```python
from build123d import *

# Parameters (mm, degrees)
SKETCH_1_R          = 15
EXTRUDE_1_DEPTH     = 20
SKETCH_10_R         = 10
EXTRUDE_10_DEPTH    = 14
SKETCH_11_R         = 10
EXTRUDE_11_DEPTH    = 14
SKETCH_12_W         = 12
SKETCH_12_H         = 50
EXTRUDE_12_DEPTH    = 10
SKETCH_13_W         = 80
SKETCH_13_H         = 12
EXTRUDE_13_DEPTH    = 10
SKETCH_14_R         = 5
CUT_EXTRUDE_1_DEPTH = 111
SKETCH_15_R         = 4
CUT_EXTRUDE_2_DEPTH = 111
SKETCH_16_R         = 7
CUT_EXTRUDE_3_DEPTH = 111
SKETCH_17_W         = 3
SKETCH_17_H         = 4
CUT_EXTRUDE_4_DEPTH = 111


with BuildPart() as part:
    # Sketch 1 → Extrude 1 (new body)
    with BuildSketch(Plane.XY.offset(-10)):
        Circle(SKETCH_1_R)
    extrude(amount=EXTRUDE_1_DEPTH)



with BuildPart() as body_2:
    # Sketch 10 → Extrude 10 (new body)
    with BuildSketch(Plane.XY.offset(-10)):
        with Locations((0, 50)):
            Circle(SKETCH_10_R)
    extrude(amount=EXTRUDE_10_DEPTH)


with BuildPart() as body_3:
    # Sketch 11 → Extrude 11 (new body)
    with BuildSketch(Plane.XY.offset(-10)):
        with Locations((80, 0)):
            Circle(SKETCH_11_R)
    extrude(amount=EXTRUDE_11_DEPTH)


with BuildPart() as part_1:
    add(part.part)

    add(body_2.part)  # Extrude 12 merges body 2
    # Sketch 12 → Extrude 12 (add)
    with BuildSketch(Plane.XY.offset(-10)):
        with Locations((0, 25)):
            Rectangle(SKETCH_12_W, SKETCH_12_H)
    extrude(amount=EXTRUDE_12_DEPTH)


    add(body_3.part)  # Extrude 13 merges body 3
    # Sketch 13 → Extrude 13 (add)
    with BuildSketch(Plane.XY.offset(-10)):
        with Locations((40, 0)):
            Rectangle(SKETCH_13_W, SKETCH_13_H)
    extrude(amount=EXTRUDE_13_DEPTH)

    # Sketch 14 → Cut-Extrude 1 (cut, through all)
    with BuildSketch(Plane.XY.offset(-10)):
        with Locations((0, 50)):
            Circle(SKETCH_14_R)
    extrude(amount=CUT_EXTRUDE_1_DEPTH, mode=Mode.SUBTRACT)

    # Sketch 15 → Cut-Extrude 2 (cut, through all)
    with BuildSketch(Plane.XY.offset(-10)):
        with Locations((80, 0)):
            Circle(SKETCH_15_R)
    extrude(amount=CUT_EXTRUDE_2_DEPTH, mode=Mode.SUBTRACT)

    # Sketch 16 → Cut-Extrude 3 (cut, through all)
    with BuildSketch(Plane.XY.offset(-10)):
        Circle(SKETCH_16_R)
    extrude(amount=CUT_EXTRUDE_3_DEPTH, mode=Mode.SUBTRACT)

    # Sketch 17 → Cut-Extrude 4 (cut, through all)
    with BuildSketch(Plane.XY.offset(-10)):
        with Locations((-7.5, 0)):
            Rectangle(SKETCH_17_W, SKETCH_17_H)
    extrude(amount=CUT_EXTRUDE_4_DEPTH, mode=Mode.SUBTRACT)


solid = part_1.part
```
Geometry: final body of the model. Coordinates: model frame, mm. A direction names the side the tool comes from. Coordinates: 2 decimals unless noted, no trailing zeros. Order: outer loops, then holes, each group sorted by start corner. A loop starts at its lowest first (then second) coordinate and runs counter-clockwise, first axis right, second up. Notation, with made-up numbers: (51.5, -29) - (61.5, -29) arc R19 cw to (61.5, -18) - close; hole circle Ø3 at (47, 48.25). An arc over 180 degrees is marked (long way). Return JSON: item names as keys, results as strings. Group by question number.
1. Cut plane D-D (z = -5.75). Output: boundary loops of the cut face in (x, y).
2. Cut plane A-A (x = 80). Output: boundary loops of the cut face in (y, z).
3. Pin query (flat end, axial travel): pin 1 (5 mm diameter, centred on x = 42, z = -4, fed in from +Y); pin 2 (1.1 mm diameter, centred on x = -7.5, z = -2.5, fed in from +Y); pin 3 (3 mm diameter, centred on y = 27, z = -4, fed in from +X). Return the tip coordinate at first contact, or that it passes through.
4. Pull-direction query (Y, two-part tool) for faces 6 (the face through (42, 6, -5)), 7 (the face through (76, 0, -3)), 8 (the face through (22, 0, -10)), 9 (the face through (42, -6, -5)); classes: pulls with the +Y half, pulls with the -Y half, needs draft (parallel to the pull), parting line crosses it, or undercut.
5. Material intervals for line 1 along X through (y, z) = (0, -2); line 2 along Y through (x, z) = (0, 0.75); line 3 along X through (y, z) = (50, -1), sorted ascending. Write a range as [from, to].
6. Cut plane C-C (z = 2.5). Output: boundary loops of the cut face in (x, y).
7. Cut plane B-B (y = 50). Output: boundary loops of the cut face in (x, z).
8. Set-up query: faces 1 (the face through (-8, -2, 0)), 2 (the face through (-5, 48, 4)), 3 (the face through (84.3, 0.1, 4)), 4 (the face through (-12, -9, 0)), 5 (the face through (6, 28, -5)). Return all of +Z, -Z, +X, -X, +Y, -Y with unobstructed straight access to the full face (end or side cutting, diameter ignored); none if empty.
Resolved:
{
 "1": {"outline": "(-6, 13.75) arc R15 ccw (long way) to (13.75, -6) - (72, -6) arc R10 ccw (long way) to (72, 6) - (13.75, 6) arc R15 ccw to (6, 13.75) - (6, 42) arc R10 ccw (long way) to (-6, 42) - close; hole (-9, -2) - (-6.71, -2) arc R7 ccw (long way) to (-6.71, 2) - (-9, 2) - close; hole circle Ø10 at (0, 50); hole circle Ø8 at (80, 0)"},
 "2": {"outline": "(-10, -10) - (-4, -10) - (-4, 4) - (-10, 4) - close; (4, -10) - (10, -10) - (10, 4) - (4, 4) - close"},
 "3": {"pin 1": "stops at y = 6", "pin 2": "stops at y = 57.19", "pin 3": "stops at x = 6"},
 "4": {"face 6": "pulls with the +Y half", "face 7": "undercut", "face 8": "needs draft", "face 9": "pulls with the -Y half"},
 "5": {"line 1": "x = [-15, -9], [7, 76], [84, 90]", "line 2": "y = [-15, -7], [7, 15], [40, 45], [55, 60]", "line 3": "x = [-10, -5], [5, 10]"},
 "6": {"outline": "circle Ø30 at (0, 0); circle Ø20 at (0, 50); circle Ø20 at (80, 0); hole (-9, -2) - (-6.71, -2) arc R7 ccw (long way) to (-6.71, 2) - (-9, 2) - close; hole circle Ø10 at (0, 50); hole circle Ø8 at (80, 0)"},
 "7": {"outline": "(-10, -10) - (-5, -10) - (-5, 4) - (-10, 4) - close; (5, -10) - (10, -10) - (10, 4) - (5, 4) - close"},
 "8": {"face 1": "+Z, -Z", "face 2": "+Z, +X, -X, +Y", "face 3": "+Z, +X, +Y, -Y", "face 4": "+Z", "face 5": "+Z, -Z, +X"}
}
